Print and shaded views of the part. All mm, measured from the part's lowest x, y and z. A direction names the side the tool comes from. Coordinates: 2 decimals unless noted, no trailing zeros. Order: outer loops, then holes, each group sorted by start corner. A loop starts at its lowest first (then second) coordinate and runs counter-clockwise, first axis right, second up. Notation, with made-up numbers: (-13, -1.5) -> (12, -1.5) arc R15 cw to (12, 18.5) -> close; hole circle Ø3 at (41, 11.5). An arc over 180 degrees is marked (long way). Write item = value, one per line. Start each with the question number.
Q1. Flat gauge pins, fed straight in: pin 1 (2.5 mm diameter, centred on x = 30.54, y = 27.37, fed in from -Z); pin 2 (8 mm diameter, centred on x = 18, z = 19, fed in from -Y); pin 3 (8 mm diameter, centred on x = 33, y = 17, fed in from +Z); pin 4 (4.5 mm diameter, centred on x = 7.56, y = 4.38, fed in from +Z). Where does each tip first touch, or does it go through?
Q2. Mould opens along Z. For the marked faces 4, 5 and 6 say: +Z half, -Z half, draft (parallel to the pull), parting line (faces both ways), or undercut.
Q3. Cut at D-D, the plane x = 10.5. List the corners of the cut face in (y, z).
Q4. Cut at A-A, the plane x = 19.05. Give the number of separate pieces and of enclosed holes in the cut face, plus the area to 3 significant figures.
Q5. Wall check: line 1 (X direction, y = 41.5, z = 22); line 2 (Y direction, x = 19, z = 2) (1 decimal); line 3 (X direction, y = 15, z = 6) (1 decimal). Give the ranges that are in metal, low to high. Write a range as from..to.
Q6. 3-axis set-ups, long thin cutter, end or side, ignore diameter. For the marked faces 1, 2 and 3: which of +Z, -Z, +X, -X, +Y, -Y reach the whole face in a straight line?
Q7. Cut at B-B, the plane y = 39. List the corners of the cut face in (x, z).
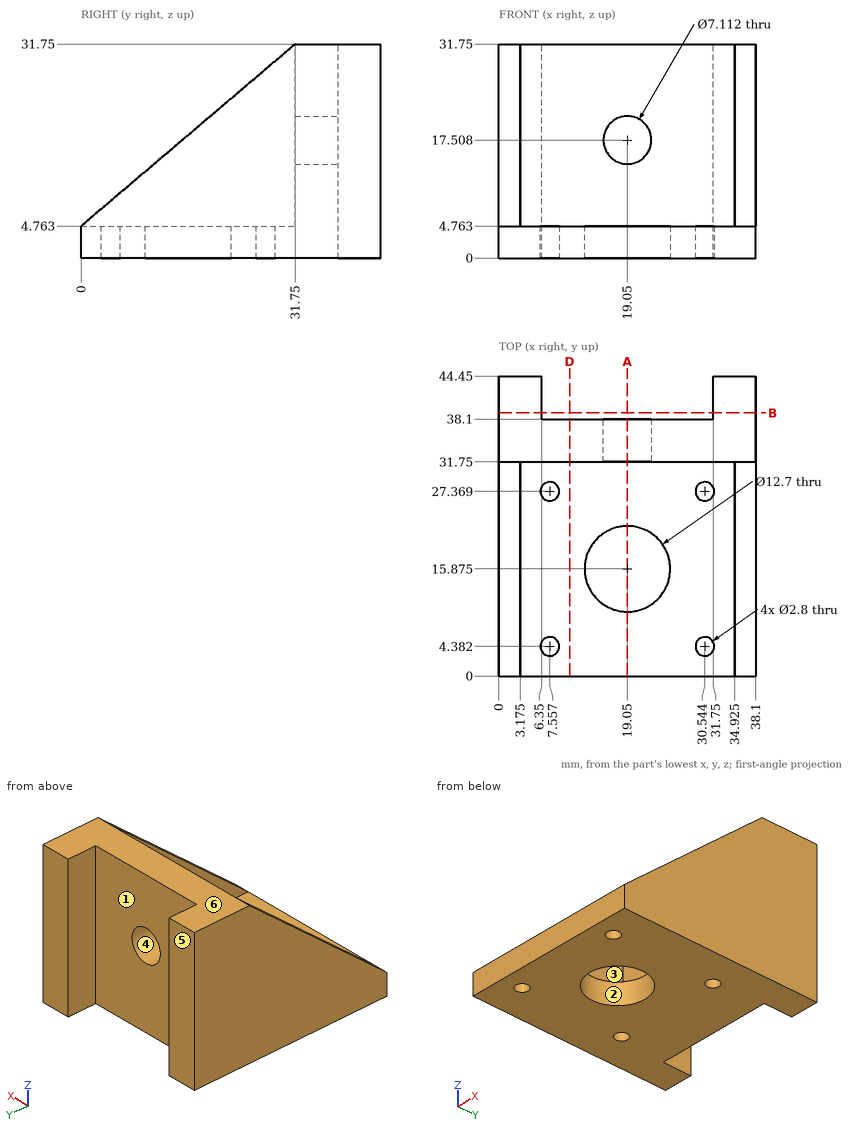
Here are the results:
q1.pin_1 = through
q1.pin_2 = 31.75
q1.pin_3 = 22.19
q1.pin_4 = 4.76
q2.face_4 = undercut
q2.face_5 = draft
q2.face_6 = +Z half
q3.outline = (0, 0) -> (38.1, 0) -> (38.1, 31.75) -> (31.75, 31.75) -> (31.75, 4.76) -> (0, 4.76) -> close
q4.separate_pieces = 3
q4.enclosed_holes = 0
q4.area = 247 mm²
q5.line_1 = 0..6.35, 31.75..38.1
q5.line_2 = 0..9.5, 22.2..38.1
q5.line_3 = 0..3.2, 34.9..38.1
q6.face_1 = +Z, -Z, +Y
q6.face_2 = +Z, -Z
q6.face_3 = +Z, -Y
q7.outline = (0, 0) -> (6.35, 0) -> (6.35, 31.75) -> (0, 31.75) -> close; (31.75, 0) -> (38.1, 0) -> (38.1, 31.75) -> (31.75, 31.75) -> close
